from build123d import *

# Parameters (mm, degrees)
SKETCH1_W           = 72
SKETCH1_H           = 5
BOSS_EXTRUDE1_DEPTH = 2
SKETCH3_R           = 0.75
CUT_EXTRUDE2_DEPTH  = 2
SKETCH4_W           = 10
SKETCH4_H           = 5
BOSS_EXTRUDE2_DEPTH = 2
SKETCH5_R           = 0.75
CUT_EXTRUDE4_DEPTH  = 2
SKETCH6_W           = 10
SKETCH6_H           = 5
BOSS_EXTRUDE3_DEPTH = 2
SKETCH7_R           = 0.75
CUT_EXTRUDE5_DEPTH  = 2


with BuildPart() as part:
    # Sketch1 → Boss-Extrude1 (new body)
    with BuildSketch(Plane.XY):
        with Locations((36, 2.5)):
            Rectangle(SKETCH1_W, SKETCH1_H)
    extrude(amount=BOSS_EXTRUDE1_DEPTH)

    # Sketch3 → Cut-Extrude2 (cut)
    with BuildSketch(Plane.XY):
        with Locations((42, 2.5)):
            Circle(SKETCH3_R)
        with Locations((54, 2.5)):
            Circle(SKETCH3_R)
        with Locations((66, 2.5)):
            Circle(SKETCH3_R)
        with Locations((30, 2.5)):
            Circle(SKETCH3_R)
        with Locations((18.06024044, 2.463599586)):
            Circle(SKETCH3_R)
        with Locations((6, 2.5)):
            Circle(SKETCH3_R)
    extrude(amount=CUT_EXTRUDE2_DEPTH, mode=Mode.SUBTRACT)

    # Sketch4 → Boss-Extrude2 (add)
    with BuildSketch(Plane(origin=(72, 0, 0), x_dir=(0, 0, -1), z_dir=(1, 0, 0))):
        with Locations((3, 2.5)):
            Rectangle(SKETCH4_W, SKETCH4_H)
    extrude(amount=BOSS_EXTRUDE2_DEPTH)

    # Sketch5 → Cut-Extrude4 (cut)
    with BuildSketch(Plane(origin=(72, 0, 0), x_dir=(0, 0, -1), z_dir=(1, 0, 0))):
        with Locations((3, 2.5)):
            Circle(SKETCH5_R)
    extrude(amount=CUT_EXTRUDE4_DEPTH, mode=Mode.SUBTRACT)

    # Sketch6 → Boss-Extrude3 (add)
    with BuildSketch(Plane.ZY):
        with Locations((-3, 2.5)):
            Rectangle(SKETCH6_W, SKETCH6_H)
    extrude(amount=BOSS_EXTRUDE3_DEPTH)

    # Sketch7 → Cut-Extrude5 (cut)
    with BuildSketch(Plane.ZY):
        with Locations((-3, 2.5)):
            Circle(SKETCH7_R)
    extrude(amount=CUT_EXTRUDE5_DEPTH, mode=Mode.SUBTRACT)


solid = part.part
The model under review builds one solid part; all positions refer to its coordinate system, in mm. A direction names the side the tool comes from. Coordinates: 2 decimals unless noted, no trailing zeros. Write each loop counter-clockwise with the first axis right and the second up, starting at its lowest first coordinate (ties: lowest second). Pieces come first, ordered by that corner, then holes. Notation, with made-up numbers: (-33.75, 30) - (-15.75, 30) arc R18 cw to (-15.75, 55) - close; hole circle Ø11 at (78, 64). An arc over 180 degrees is marked (long way). Answer as a JSON object with one key per item and string values. Group by question number.
1. Mouldability with a two-part tool opening along Z and no side actions: class faces 3 (the face through (27.7, 5, 0.3)), 4 (the face through (72.986, 2.044, -2.405)), 5 (the face through (-0.986, 2.044, -3.595)), 6 (the face through (35, 3, 0)) as pulls with the +Z half, pulls with the -Z half, needs draft (parallel to the pull), parting line crosses it, or undercut.
2. To check wall thickness, follow probe 1 along X at (y, z) = (2.1, -5.5); probe 2 along Y at (x, z) = (30, 0.55); probe 3 along Z at (x, y) = (17.5, 4.2). State the ranges of each line that lie inside material, in increasing order.
3. Clearance check with flat-ended pins moving along their axes: pin 1 Ø1.5 at (x, z) = (38.5, -1) entering from +Y; pin 2 Ø2.5 at (x, y) = (39, 1.5) entering from -Z; pin 3 Ø1.5 at (y, z) = (2.5, -3.5) entering from +X. State where each tip first meets the part, or that it passes through.
4. Add section C-C (z = -3). Give the boundary of the cut face in (x, y), plus the area to 3 significant figures.
5. Add section B-B (z = -6). Give the boundary of the cut face in (x, y).
6. Machinability: for faces 1 (the face through (72, 3, -4)), 2 (the face through (65.25, 2.53, 0.99)), which of the approach directions +Z, -Z, +X, -X, +Y, -Y give a long, thin tool a straight path to every point of the face, cutting with its end or side? Answer none if there is none.
7. Add section D-D (y = 4.05). Give the boundary of the cut face in (x, z).
8. Add section A-A (x = 66). Give the boundary of the cut face in (y, z), plus the area to 3 significant figures.
Findings:
{
 "1": {"face 3": "needs draft", "face 4": "undercut", "face 5": "undercut", "face 6": "pulls with the -Z half"},
 "2": {"probe 1": "-2 to 0, 72 to 74", "probe 2": "0 to 1.75, 3.25 to 5", "probe 3": "0 to 2"},
 "3": {"pin 1": "through", "pin 2": "z = 0", "pin 3": "x = 74"},
 "4": {"outline": "(-2, 0) - (0, 0) - (0, 1.75) - (-2, 1.75) - close; (-2, 3.25) - (0, 3.25) - (0, 5) - (-2, 5) - close; (72, 0) - (74, 0) - (74, 1.75) - (72, 1.75) - close; (72, 3.25) - (74, 3.25) - (74, 5) - (72, 5) - close", "area": "14.0 mm²"},
 "5": {"outline": "(-2, 0) - (0, 0) - (0, 5) - (-2, 5) - close; (72, 0) - (74, 0) - (74, 5) - (72, 5) - close"},
 "6": {"face 1": "-Z, +Y, -Y", "face 2": "+Z, -Z"},
 "7": {"outline": "(-2, -8) - (0, -8) - (0, 0) - (72, 0) - (72, -8) - (74, -8) - (74, 2) - (-2, 2) - close"},
 "8": {"outline": "(0, 0) - (1.75, 0) - (1.75, 2) - (0, 2) - close; (3.25, 0) - (5, 0) - (5, 2) - (3.25, 2) - close", "area": "7.00 mm²"}
}
